```python
from build123d import *

# Parameters (mm, degrees)
EXTRUDE_1_DEPTH          = 24
CUT_EXTRUDE_2_REACH      = 50.6
SKETCH_3_R               = 3.15
SKETCH_4_W               = 18.4
SKETCH_4_H               = 17.2
SKETCH_4_H_2             = 10
EXTRUDE_2_DEPTH          = 10
SKETCH_4_3_W             = 18.4
SKETCH_4_3_H             = 17.2
CUT_EXTRUDE_4_DEPTH      = 5
SKETCH_4_5_W             = 18.4
SKETCH_4_5_H             = 10
CUT_EXTRUDE_6_DEPTH      = 2
SKETCH_2_R               = 20.05
SKETCH_2_R_2             = 1.6
EXTRUDE_3_DEPTH          = 5
SKETCH_7_R               = 1.6
CUT_EXTRUDE_7_DEPTH      = 77.51774304
SKETCH_8_R               = 3
CUT_EXTRUDE_8_DEPTH      = 3.2
CUT_EXTRUDE_8_DEPTH_BACK = 3.2


with BuildPart() as part:
    # 草圖1 → 填料-伸長1 (new, symmetric)
    with BuildSketch(Plane.XY):
        Polygon((0, 0), (0, 33), (26.4, 33), (26.4, 0), (22.4, 0), (22.4, 27.2), (4, 27.2), (4, 0), align=None)
    extrude(amount=EXTRUDE_1_DEPTH, both=True)

    # 除料-伸長2: up to this face of the body (flat: up to its plane)
    cut_extrude_2_end = Plane(part.part.faces().sort_by_distance((0, 16.5, 0))[0])
    # 草圖3 → 除料-伸長2 (cut, up to the picked face)
    with BuildSketch(Plane(origin=(26.4, 0, 0), x_dir=(0, 0, -1), z_dir=(1, 0, 0)), mode=Mode.PRIVATE) as cut_extrude_2_sk1:
        with Locations(Location((0, 6, 0), (0, 0, 90))):
            Circle(SKETCH_3_R)
    cut_extrude_2_tool1 = split(extrude(cut_extrude_2_sk1.sketch, amount=-CUT_EXTRUDE_2_REACH, mode=Mode.PRIVATE), bisect_by=cut_extrude_2_end, keep=Keep.BOTH, mode=Mode.PRIVATE)
    # 草圖3 → 除料-伸長2 (cut, up to the picked face)
    with BuildSketch(Plane(origin=(26.4, 0, 0), x_dir=(0, 0, -1), z_dir=(1, 0, 0)), mode=Mode.PRIVATE) as cut_extrude_2_sk2:
        with Locations(Location((15, 6, 0), (0, 0, 90))):
            Circle(SKETCH_3_R)
    cut_extrude_2_tool2 = split(extrude(cut_extrude_2_sk2.sketch, amount=-CUT_EXTRUDE_2_REACH, mode=Mode.PRIVATE), bisect_by=cut_extrude_2_end, keep=Keep.BOTH, mode=Mode.PRIVATE)
    # 草圖3 → 除料-伸長2 (cut, up to the picked face)
    with BuildSketch(Plane(origin=(26.4, 0, 0), x_dir=(0, 0, -1), z_dir=(1, 0, 0)), mode=Mode.PRIVATE) as cut_extrude_2_sk3:
        with Locations(Location((-15, 6, 0), (0, 0, 90))):
            Circle(SKETCH_3_R)
    cut_extrude_2_tool3 = split(extrude(cut_extrude_2_sk3.sketch, amount=-CUT_EXTRUDE_2_REACH, mode=Mode.PRIVATE), bisect_by=cut_extrude_2_end, keep=Keep.BOTH, mode=Mode.PRIVATE)
    add(cut_extrude_2_tool1.solids().sort_by(Axis((26.4, 6, 0), (-1, 0, 0)))[0], mode=Mode.SUBTRACT)
    add(cut_extrude_2_tool2.solids().sort_by(Axis((26.4, 6, -15), (-1, 0, 0)))[0], mode=Mode.SUBTRACT)
    add(cut_extrude_2_tool3.solids().sort_by(Axis((26.4, 6, 15), (-1, 0, 0)))[0], mode=Mode.SUBTRACT)

    # 草圖4 → 填料-伸長2 (add)
    with BuildSketch(Plane(origin=(0, 0, -24), x_dir=(-1, 0, 0), z_dir=(0, 0, -1))):
        Polygon((-4, 27.2), (-4, 0), (0, 0), (0, 33), (-26.4, 33), (-26.4, 0), (-22.4, 0), (-22.4, 27.2), align=None)
        with Locations((-13.2, 18.6)):
            Rectangle(SKETCH_4_W, SKETCH_4_H)
        with Locations((-13.2, 5)):
            Rectangle(SKETCH_4_W, SKETCH_4_H_2)
    extrude(amount=EXTRUDE_2_DEPTH)

    # 草圖4<3> → 除料-伸長4 (cut)
    with BuildSketch(Plane(origin=(0, 0, -24), x_dir=(-1, 0, 0), z_dir=(0, 0, -1))):
        with Locations((-13.2, 18.6)):
            Rectangle(SKETCH_4_3_W, SKETCH_4_3_H)
    extrude(amount=CUT_EXTRUDE_4_DEPTH, mode=Mode.SUBTRACT)

    # 草圖4<5> → 除料-伸長6 (cut)
    with BuildSketch(Plane(origin=(0, 0, -24), x_dir=(-1, 0, 0), z_dir=(0, 0, -1))):
        with Locations((-13.2, 5)):
            Rectangle(SKETCH_4_5_W, SKETCH_4_5_H)
    extrude(amount=CUT_EXTRUDE_6_DEPTH, mode=Mode.SUBTRACT)

    # 草圖2 → 填料-伸長3 (add)
    with BuildSketch(Plane(origin=(60.4, 53.6, -34), x_dir=(0, -1, 0), z_dir=(0, 0, 1))):
        with Locations((29.6, -47.2)):
            Circle(SKETCH_2_R)
        with Locations(Location((13.1, -47.2, 0), (0, 0, 90))):
            Circle(SKETCH_2_R_2, mode=Mode.SUBTRACT)
        with Locations((37.85, -32.910580838)):
            Circle(SKETCH_2_R_2, mode=Mode.SUBTRACT)
        with Locations((37.85, -61.489419162)):
            Circle(SKETCH_2_R_2, mode=Mode.SUBTRACT)
    extrude(amount=EXTRUDE_3_DEPTH)

    # 草圖7 → 除料-伸長7 (cut, through all)
    with BuildSketch(Plane.XY.offset(-29)):
        with Locations(Location((27.489419162, 15.75, 0), (0, 0, 227.087006542))):
            Circle(SKETCH_7_R)
        with Locations(Location((-1.089419162, 15.75, 0), (0, 0, 312.912993458))):
            Circle(SKETCH_7_R)
    extrude(amount=-CUT_EXTRUDE_7_DEPTH, mode=Mode.SUBTRACT)

    # 草圖8 → 除料-伸長8 (cut, two sides)
    with BuildSketch(Plane.XY.offset(-29)) as cut_extrude_8_sk:
        with Locations(Location((-1.089419162, 15.75, 0), (0, 0, 68.706857297))):
            Circle(SKETCH_8_R)
        with Locations(Location((27.489419162, 15.75, 0), (0, 0, 248.706857297))):
            Circle(SKETCH_8_R)
        with Locations((13.2, 40.5)):
            Circle(SKETCH_8_R)
    extrude(amount=CUT_EXTRUDE_8_DEPTH, mode=Mode.SUBTRACT)
    extrude(cut_extrude_8_sk.sketch, amount=-CUT_EXTRUDE_8_DEPTH_BACK, mode=Mode.SUBTRACT)


solid = part.part
```
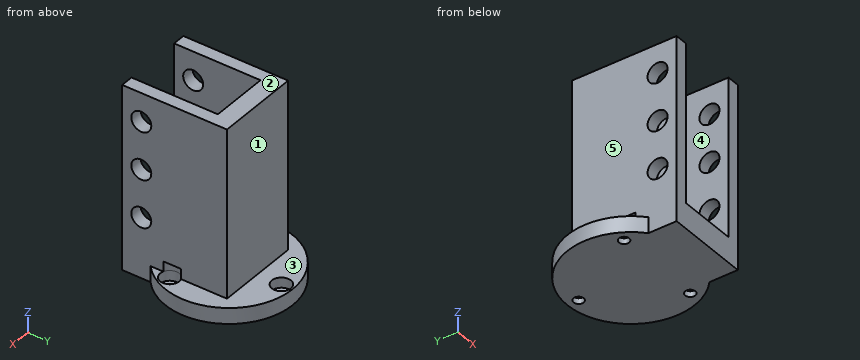
The listing builds one solid part. Answer for the finished solid, in the listing's coordinates (mm). Face numbers are marked on the shaded views. A direction names the side the tool comes from. Round coordinates to 2 decimals unless told otherwise and drop trailing zeros. Order: outer loops, then holes, each group sorted by start corner. A loop starts at its lowest first (then second) coordinate and runs counter-clockwise, first axis right, second up. Notation, with made-up numbers: (84, 34.25) - (107, 34.25) arc R16 cw to (107, 58.25) - close; hole circle Ø11 at (50.5, -13.75). An arc over 180 degrees is marked (long way). Put each result on its own line as item: value. Start each with the question number.
(1) Given P1, Ø2, axis at x = 4, z = -17.5, coming from the +Y side; P2, Ø5, axis at x = 28.5, y = 16.5, coming from the +Z side; P3, Ø7, axis at x = 13.2, y = 40.5, coming from the +Z side; P4, Ø4, axis at y = 9.5, z = 4.5, coming from the -X side, each flat-ended and moving along its own axis, determine where each tip first touches the part or whether it passes through.
(2) Find section D-D (y = 24). Give the vertices of the cut face in (x, z).
(3) Find section A-A (z = -15). Give the vertices of the cut face in (x, y), plus the area to 3 significant figures.
(4) For the marked faces 1 and 2, determine the directions among +Z, -Z, +X, -X, +Y, -Y from which every point of the face is accessible in a straight line to the end or side of a thin tool.
(5) Find section C-C (x = 13.2). Give the vertices of the cut face in (y, z).
(6) Determine the mould class of the marked faces 3, 4 and 5 for opening direction X: released by +X, released by -X, zero draft, split by the parting line, or undercut.
(7) Straight lines are drawn through the part: probe 1 along Z at (x, y) = (24, 6); probe 2 along X at (y, z) = (17.5, -19.5); probe 3 along Z at (x, y) = (25, 5). For each, find the intervals that lie inside material, in ascending order. Write a range as from..to.
(8) Find section B-B (y = 6). State how many separate pieces and enclosed holes the cut face has, plus the area to 3 significant figures.
Reply:
1. P1: y = 33
1. P2: z = 24
1. P3: z = -29
1. P4: x = 0
2. outline: (-6.85, -34) - (33.25, -34) - (33.25, -29) - (26.4, -29) - (26.4, 24) - (22.4, 24) - (22.4, -29) - (4, -29) - (4, 24) - (0, 24) - (0, -29) - (-6.85, -29) - close
3. outline: (0, 0) - (4, 0) - (4, 2.85) - (0, 2.85) - close; (0, 9.15) - (4, 9.15) - (4, 27.2) - (22.4, 27.2) - (22.4, 9.15) - (26.4, 9.15) - (26.4, 33) - (0, 33) - close; (22.4, 0) - (26.4, 0) - (26.4, 2.85) - (22.4, 2.85) - close
3. area: 320 mm^2
4. face 1: +Z, +X, -X, +Y
4. face 2: +Z, +X, -X, +Y, -Y
5. outline: (0, -34) - (38.9, -34) - (38.9, -32.2) - (37.5, -32.2) - (37.5, -29) - (33, -29) - (33, 24) - (27.2, 24) - (27.2, -29) - (10, -29) - (10, -26) - (0, -26) - close; (42.1, -34) - (44.05, -34) - (44.05, -29) - (43.5, -29) - (43.5, -32.2) - (42.1, -32.2) - close
6. face 3: zero draft
6. face 4: undercut
6. face 5: released by -X
7. probe 1: -34..-18.15, -11.85..-3.15, 3.15..11.85, 18.15..24
7. probe 2: 0..4, 22.4..26.4
7. probe 3: -34..-17.99, -12.01..-2.99, 2.99..12.01, 17.99..24
8. separate pieces: 7
8. enclosed holes: 0
8. area: 460 mm^2
